Here's how the part is built. I have some questions about the finished solid (model axes, mm). A direction names the side the tool comes from. Round coordinates to 2 decimals unless told otherwise and drop trailing zeros. Order: outer loops, then holes, each group sorted by start corner. A loop starts at its lowest first (then second) coordinate and runs counter-clockwise, first axis right, second up. Notation, with made-up numbers: (78.5, 56.5) -> (111.5, 56.5) arc R24 ccw to (111.5, 95.5) -> close; hole circle Ø10 at (-39.5, -2). An arc over 180 degrees is marked (long way). Use a Markdown table: item, result. Add a question column.
from build123d import *

# Parameters (mm, degrees)
SKETCH1_W               = 8
SKETCH1_H               = 8
SKETCH1_R               = 1.65
BOSS_EXTRUDE1_DEPTH     = 3
BOSS_EXTRUDE2_DEPTH     = 22
SKETCH3_R               = 13
CUT_EXTRUDE1_DEPTH      = 92.431135288
CUT_EXTRUDE3_DEPTH      = 3
SKETCH6_R               = 1.65
SKETCH6_W               = 51.3
SKETCH6_H               = 32.3
CUT_EXTRUDE4_DEPTH      = 93.198983183
BOSS_EXTRUDE4_DEPTH     = 25
CUT_EXTRUDE5_DEPTH      = 93.198983183
SKETCH10_W              = 12
SKETCH10_H              = 12
CUT_EXTRUDE6_DEPTH      = 93.198983183
SKETCH11_W              = 5
SKETCH11_H              = 5
CUT_EXTRUDE7_DEPTH      = 10
CUT_EXTRUDE8_DEPTH      = 93.198983183
CUT_EXTRUDE8_DEPTH_BACK = 93.198983183


# Read off the part's stored shape, not the designer's step: Cut-Extrude3
with BuildPart() as part:
    # Sketch1 → Boss-Extrude1 (new body)
    # profile 1 of 4: a face of its own
    with BuildSketch(Plane(origin=(0, 0, 0), x_dir=(1, 0, 0), z_dir=(0, 1, 0))):
        with BuildLine():
            Line((-18.5, 69.116947994), (-18.5, 4))
            Line((-18.5, 4), (-18.5, -4))
            Line((-18.5, -4), (-18.5, -65.642897559))
            ThreePointArc((-18.5, -65.642897559), (14.755653403, -66.584613032), (44.5, -51.681621492))
            Line((44.5, -51.681621492), (44.5, -28))
            Line((44.5, -28), (44.5, -20))
            Line((44.5, -20), (44.5, 20))
            Line((44.5, 20), (44.5, 28))
            Line((44.5, 28), (44.5, 55))
            Line((44.5, 55), (44.5, 56.028140251))
            ThreePointArc((44.5, 56.028140251), (14.554354058, 70.054073957), (-18.5, 69.116947994))
        make_face()
    # profile 2 of 4: a face of its own
    with BuildSketch(Plane(origin=(0, 0, 0), x_dir=(1, 0, 0), z_dir=(0, 1, 0))):
        with Locations((-22.5, 0)):
            Rectangle(SKETCH1_W, SKETCH1_H)
        with Locations(Location((-22.5, 0, 0), (0, 0, 270))):
            Circle(SKETCH1_R, mode=Mode.SUBTRACT)
    # profile 3 of 4: a face of its own
    with BuildSketch(Plane(origin=(0, 0, 0), x_dir=(1, 0, 0), z_dir=(0, 1, 0))):
        with Locations((48.5, -24)):
            Rectangle(SKETCH1_W, SKETCH1_H)
        with Locations(Location((48.5, -24, 0), (0, 0, 270))):
            Circle(SKETCH1_R, mode=Mode.SUBTRACT)
    # profile 4 of 4: a face of its own
    with BuildSketch(Plane(origin=(0, 0, 0), x_dir=(1, 0, 0), z_dir=(0, 1, 0))):
        with Locations((48.5, 24)):
            Rectangle(SKETCH1_W, SKETCH1_H)
        with Locations(Location((48.5, 24, 0), (0, 0, 270))):
            Circle(SKETCH1_R, mode=Mode.SUBTRACT)
    extrude(amount=BOSS_EXTRUDE1_DEPTH)

    # Sketch2 → Boss-Extrude2 (add)
    with BuildSketch(Plane(origin=(0, 3, 0), x_dir=(1, 0, 0), z_dir=(0, 1, 0))):
        with BuildLine():
            Line((44.5, -42.522376462), (44.5, 42.522376462))
            ThreePointArc((44.5, 42.522376462), (42.065161183, 44.932446124), (39.5, 47.203310265))
            Line((39.5, 47.203310265), (39.5, -47.203310265))
            ThreePointArc((39.5, -47.203310265), (42.065161183, -44.932446124), (44.5, -42.522376462))
        make_face()
    extrude(amount=BOSS_EXTRUDE2_DEPTH)

    # Sketch3 → Cut-Extrude1 (cut, through all)
    with BuildSketch(Plane(origin=(0, 3, 0), x_dir=(1, 0, 0), z_dir=(0, 1, 0))):
        with Locations((-30, -20.7)):
            Circle(SKETCH3_R)
    extrude(amount=-CUT_EXTRUDE1_DEPTH, mode=Mode.SUBTRACT)

    # Cut-Extrude3 outline → Cut-Extrude3 (cut)
    with BuildSketch(Plane(origin=(0, 0, 0), x_dir=(1, 0, 0), z_dir=(0, 1, 0))):
        with BuildLine():
            Line((44.5, -51.681621492), (44.5, -42.522376462))
            ThreePointArc((44.5, -42.522376462), (42.879948374, -44.155549226), (41.2, -45.727043421))
            Line((41.2, -45.727043421), (41.2, -54.348873033))
            ThreePointArc((41.2, -54.348873033), (42.870748276, -53.040917623), (44.5, -51.681621492))
        make_face()
        with BuildLine():
            ThreePointArc((41.2, 45.727043421), (42.879948374, 44.155549226), (44.5, 42.522376462))
            Line((44.5, 42.522376462), (44.5, 56.028140251))
            ThreePointArc((44.5, 56.028140251), (42.867784957, 57.286608495), (41.2, 58.497542683))
            Line((41.2, 58.497542683), (41.2, 45.727043421))
        make_face()
        with BuildLine():
            ThreePointArc((-18.5, -65.642897559), (-16.85525465, -66.084343007), (-15.2, -66.484584679))
            Line((-15.2, -66.484584679), (-15.2, -59.091509852))
            ThreePointArc((-15.2, -59.091509852), (-16.856674237, -58.640421812), (-18.5, -58.142897559))
            Line((-18.5, -58.142897559), (-18.5, -65.642897559))
        make_face()
    extrude(amount=CUT_EXTRUDE3_DEPTH, mode=Mode.SUBTRACT)

    # Sketch6 → Cut-Extrude4 (cut, through all)
    with BuildSketch(Plane(origin=(0, 0, 0), x_dir=(1, 0, 0), z_dir=(0, 1, 0))):
        with Locations(Location((-9.25, 44.6, 0), (0, 0, 90))):
            Circle(SKETCH6_R)
        with Locations(Location((-9.25, 4.6, 0), (0, 0, 90))):
            Circle(SKETCH6_R)
        with Locations(Location((30.75, 4.6, 0), (0, 0, 90))):
            Circle(SKETCH6_R)
        with Locations(Location((30.75, 44.6, 0), (0, 0, 90))):
            Circle(SKETCH6_R)
        with Locations(Location((-9.25, -4.6, 0), (0, 0, 90))):
            Circle(SKETCH6_R)
        with Locations(Location((30.75, -4.6, 0), (0, 0, 90))):
            Circle(SKETCH6_R)
        with Locations(Location((30.75, -44.6, 0), (0, 0, 90))):
            Circle(SKETCH6_R)
        with Locations(Location((-9.25, -44.6, 0), (0, 0, 90))):
            Circle(SKETCH6_R)
        with Locations((10.75, 23.5)):
            Rectangle(SKETCH6_W, SKETCH6_H)
        with Locations((10.75, -23.5)):
            Rectangle(SKETCH6_W, SKETCH6_H)
    extrude(amount=CUT_EXTRUDE4_DEPTH, mode=Mode.SUBTRACT)

    # Sketch8 → Boss-Extrude4 (add)
    with BuildSketch(Plane(origin=(0, 0, 0), x_dir=(1, 0, 0), z_dir=(0, 1, 0))):
        with BuildLine():
            Line((41, 58.637893039), (41, 54.93725967))
            ThreePointArc((41, 54.93725967), (14.207393879, 67.061557238), (-15.2, 66.843567379))
            Line((-15.2, 66.843567379), (-15.2, 69.916825586))
            ThreePointArc((-15.2, 69.916825586), (14.078834464, 70.151186164), (41, 58.637893039))
        make_face()
    extrude(amount=BOSS_EXTRUDE4_DEPTH)

    # Sketch9 → Cut-Extrude5 (cut, through all)
    with BuildSketch(Plane(origin=(0, 0, 0), x_dir=(1, 0, 0), z_dir=(0, 1, 0))):
        with BuildLine():
            Line((-18.5, 58.703939391), (-18.5, 74.933190401))
            Line((-18.5, 74.933190401), (-15.2, 74.933190401))
            Line((-15.2, 74.933190401), (-15.2, 59.643629165))
            ThreePointArc((-15.2, 59.643629165), (-16.856549297, 59.196784083), (-18.5, 58.703939391))
        make_face()
    extrude(amount=CUT_EXTRUDE5_DEPTH, mode=Mode.SUBTRACT)

    # Sketch10 → Cut-Extrude6 (cut, through all)
    with BuildSketch(Plane(origin=(0, 0, 0), x_dir=(1, 0, 0), z_dir=(0, 1, 0))):
        with Locations((-4, 58)):
            Rectangle(SKETCH10_W, SKETCH10_H)
    extrude(amount=CUT_EXTRUDE6_DEPTH, mode=Mode.SUBTRACT)

    # Sketch11 → Cut-Extrude7 (cut)
    with BuildSketch(Plane(origin=(0, 3, 0), x_dir=(1, 0, 0), z_dir=(0, 1, 0))):
        with Locations((37, 0)):
            Rectangle(SKETCH11_W, SKETCH11_H)
    extrude(amount=-CUT_EXTRUDE7_DEPTH, mode=Mode.SUBTRACT)

    # Sketch13 → Cut-Extrude8 (cut, two sides: drawn at the far end of the back side and taken through both)
    with BuildSketch(Plane(origin=(0, 0, 0), x_dir=(0, 0, -1), z_dir=(1, 0, 0)).offset(-CUT_EXTRUDE8_DEPTH_BACK)):
        Polygon((55.086575096, 0), (71.55, 2.244157451), (71.55, 0), align=None)
    extrude(amount=CUT_EXTRUDE8_DEPTH + CUT_EXTRUDE8_DEPTH_BACK, mode=Mode.SUBTRACT)


solid = part.part
(1) Please list where these lines run through material, in increasing order: probe 1 along X at (y, z) = (1.55, 4.6); probe 2 along X at (y, z) = (2.3, -24); probe 3 along Y at (x, z) = (25, 42.5). Write a range as from..to.
(2) I want a section at B-B on y = 9. List the corners of the cut face in (x, z) for me, and give its area (3 significant figures).
(3) On a 3-axis mill with a long thin cutter (end or side, diameter ignored), from which of +Z, -Z, +X, -X, +Y, -Y can I reach the whole of each face in a straight line? I mean faces 4 (the flat face through (41.2, 1, 50)), 5 (the flat face through (46.7, 3, 23.9)), 6 (the flat face through (2, 2, -58)). Say none if no direction works.
(4) I want a section at A-A on x = 48.5. List the corners of the cut face in (y, z) for me, and give its area (3 significant figures).
(5) I want a section at D-D on z = 24. List the corners of the cut face in (x, y) for me, and give its area (3 significant figures).
(6) I want a section at C-C on x = 30.75. State how many separate pieces and enclosed holes the cut face has, and give its area (3 significant figures).
(7) If we mould it in two halves opening along Z, with no side actions, what happens to faces 1 (the flat face through (14, 0, 6)), 2 (the flat face through (-23, 1, 4)), 3 (the cylindrical face through (29.635, 1.479, -43.384))? For each: pulls with the +Z half, pulls with the -Z half, needs draft (parallel to the pull), parting line crosses it, or undercut.
(8) I'm going to push flat-ended pins straight in: P1, Ø1.5, axis at x = 38, y = 12, coming from the -Z side; P2, Ø8, axis at y = 15.5, z = -29, coming from the +X side; P3, Ø0.9, axis at y = 1, z = 39, coming from the -X side; P4, Ø4, axis at x = 48.5, z = 24, coming from the -Y side. Where does each tip first touch, or does it pass through?
Output:
| question | item | result |
|---|---|---|
| 1 | probe 1 | -18.5..-10.9, -7.6..29.1, 32.4..44.5 |
| 1 | probe 2 | -18.5..-14.9, 36.4..46.85, 50.15..52.5 |
| 1 | probe 3 | 0..3 |
| 2 | outline | (-15.2, -69.92) arc R71.55 ccw to (41, -58.64) -> (41, -54.94) arc R68.55 cw to (-15.2, -66.84) -> close; (39.5, -47.2) arc R61.55 ccw to (44.5, -42.52) -> (44.5, 42.52) arc R61.55 ccw to (39.5, 47.2) -> close |
| 2 | area | 627 mm² |
| 3 | face 4 | +Z, +X, +Y, -Y |
| 3 | face 5 | +Z, -Z, +X, +Y |
| 3 | face 6 | +Y, -Y |
| 4 | outline | (0, -28) -> (3, -28) -> (3, -25.65) -> (0, -25.65) -> close; (0, -22.35) -> (3, -22.35) -> (3, -20) -> (0, -20) -> close; (0, 20) -> (3, 20) -> (3, 22.35) -> (0, 22.35) -> close; (0, 25.65) -> (3, 25.65) -> (3, 28) -> (0, 28) -> close |
| 4 | area | 28.2 mm² |
| 5 | outline | (-17.43, 0) -> (-14.9, 0) -> (-14.9, 3) -> (-17.43, 3) -> close; (36.4, 0) -> (46.85, 0) -> (46.85, 3) -> (44.5, 3) -> (44.5, 25) -> (39.5, 25) -> (39.5, 3) -> (36.4, 3) -> close; (50.15, 0) -> (52.5, 0) -> (52.5, 3) -> (50.15, 3) -> close |
| 5 | area | 156 mm² |
| 6 | separate pieces | 7 |
| 6 | enclosed holes | 0 |
| 6 | area | 210 mm² |
| 7 | face 1 | needs draft |
| 7 | face 2 | pulls with the +Z half |
| 7 | face 3 | undercut |
| 8 | P1 | z = -61.09 |
| 8 | P2 | x = 44.5 |
| 8 | P3 | x = -18.5 |
| 8 | P4 | y = 0 |
